Autodesk Inventor part; units mm, degrees
ref_plane "YZ Plane" through (0, 0, 0) normal (1, 0, 0) x (0, 1, 0)
ref_plane "XZ Plane" through (0, 0, 0) normal (0, 1, 0) x (-1, 0, 0)
ref_plane "XY Plane" through (0, 0, 0) normal (0, 0, 1) x (1, 0, 0)
sketch "Sketch1" plane through (0, 0, 0) normal (0, 1, 0) x (-1, 0, 0)
  line L0 (100, 85) -> (-100, 85)
  line L1 (-100, 85) -> (-100, -85)
  line L2 (-100, -85) -> (100, -85)
  line L3 (100, -85) -> (100, 85)
  point P0 (0, 0)
  point P1 (0, 85)
  point P2 (100, 0)
  dimension "d0" = 200
  dimension "d1" = 170
extrude "Plate1" add sketch "Sketch1" along normal blind 8
sketch "Sketch2" plane through (0, 0, 0) normal (0, -1, 0) x (1, 0, 0)
  line L0 (80, 65) -> (80, -65) construction
  line L1 (-100, -85) -> (-100, 85)
  line L2 (100, 85) -> (100, -85)
  point P0 (0, 0)
  point P1 (80, 0)
  point P2 (-100, 0)
  dimension "d10" = 20
  dimension "d12" = 20
hole "Hole1" at (80, 0, 65) at (80, 0, -65) direction (0, 1, 0) diameter 17 end through all
fillet "Corner Round1" radius 6 4 edges at (100, 4, 85) (100, 4, -85) (-100, 4, -85) (-100, 4, 85)
mirror "Mirror1" about plane through (0, 0, 0) normal (1, 0, 0) of "Hole1"
equation "\"d12\" = d10"
equation "\"d8\" = Thickness"
equation "\"d2\" = Thickness"
equation "\"BendRadius\" = Thickness"
equation "\"BendReliefWidth\" = Thickness"
equation "\"BendReliefDepth\" = 0.5 * Thickness"
equation "\"CornerReliefSize\" = 4 * Thickness"
equation "\"MinimumRemnant\" = 2 * Thickness"
equation "\"TransitionRadius\" = BendRadius"
equation "\"JacobiRadiusSize\" = BendRadius"
equation "\"GapSize\" = Thickness"
properties part number "пластина нижняя соед X16"
Could you check a few things on this model? Use its own coordinates, in mm. Give positions to 0.01 mm unless a question says otherwise; leave off trailing zeros. Loops run counter-clockwise (first coordinate to the right, second up) from the corner with the lowest first, then second, coordinate; pieces in that order, holes last. Notation, with made-up numbers: (-10.75, 14) -> (-6.75, 14) arc R18 cw to (-6.75, 33) -> close; hole circle Ø4 at (-24, 70). An arc over 180 degrees is marked (long way). Return JSON: item names as keys, results as strings.
Item 1: If we section it at C-C on x = 80: List the corners of the cut face in (y, z) for me.
Geometry results:
{"outline": "(0, -85) -> (8, -85) -> (8, -73.5) -> (0, -73.5) -> close; (0, -56.5) -> (8, -56.5) -> (8, 56.5) -> (0, 56.5) -> close; (0, 73.5) -> (8, 73.5) -> (8, 85) -> (0, 85) -> close"}
Item 2: We'd pull the mould along X, two halves only. Please class faces 1 (the cylindrical face through (-98.196, 4.056, -83.289)), 2 (the flat face through (1, 4, -85)), 3 (the cylindrical face through (74.255, 4.056, 71.265)): +X half, -X half, draft (parallel to the pull), parting line (faces both ways), or undercut.
Geometry results:
{"face 1": "-X half", "face 2": "draft", "face 3": "undercut"}
Item 3: If we section it at A-A on z = -65: List the corners of the cut face in (x, y) for me.
Geometry results:
{"outline": "(-100, 0) -> (-88.5, 0) -> (-88.5, 8) -> (-100, 8) -> close; (-71.5, 0) -> (71.5, 0) -> (71.5, 8) -> (-71.5, 8) -> close; (88.5, 0) -> (100, 0) -> (100, 8) -> (88.5, 8) -> close"}
Item 4: If we section it at B-B on y = 2: List the corners of the cut face in (x, z) for me.
Geometry results:
{"outline": "(-100, -79) arc R6 ccw to (-94, -85) -> (94, -85) arc R6 ccw to (100, -79) -> (100, 79) arc R6 ccw to (94, 85) -> (-94, 85) arc R6 ccw to (-100, 79) -> close; hole circle Ø17 at (-80, -65); hole circle Ø17 at (-80, 65); hole circle Ø17 at (80, -65); hole circle Ø17 at (80, 65)"}
Item 5: I'm going to push a flat-ended pin straight in: pin 1 (13.5 mm diameter, centred on x = -80, z = -65, fed in from -Y). Where does the tip first touch, or does it pass through?
Geometry results:
{"pin 1": "passes through"}
Item 6: I need wall thicknesses on L1, parallel to X at y = 6.25, z = -65; L2, parallel to Z at x = -80, y = 3; L3, parallel to Z at x = -76, y = 3.5. Which ranges of each line are inside material? Lowest first, please. Write a range as from..to.
Geometry results:
{"L1": "x = -100..-88.5, -71.5..71.5, 88.5..100", "L2": "z = -85..-73.5, -56.5..56.5, 73.5..85", "L3": "z = -85..-72.5, -57.5..57.5, 72.5..85"}
